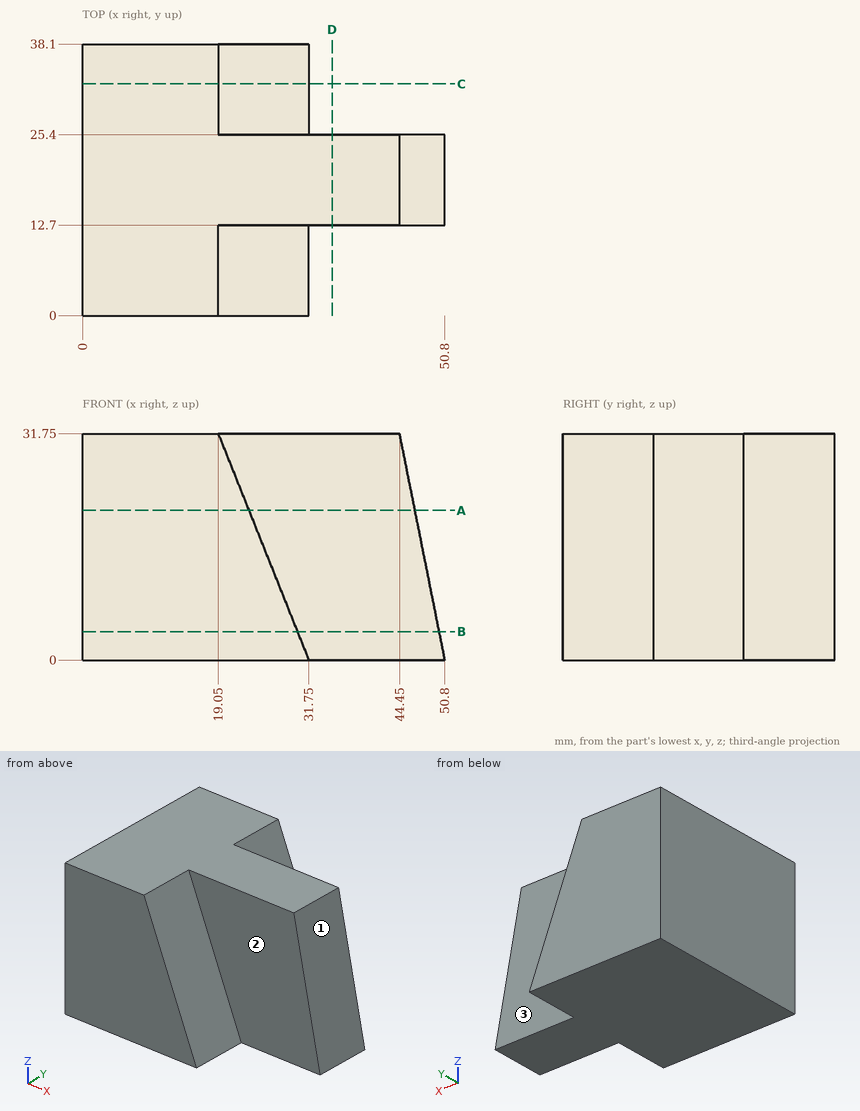
Drawing for the job (mm, zero at the part's lowest x, y, z). A direction names the side the tool comes from. Round coordinates to 2 decimals unless told otherwise and drop trailing zeros. Loops run counter-clockwise (first coordinate to the right, second up) from the corner with the lowest first, then second, coordinate; pieces in that order, holes last. Notation, with made-up numbers: (78.25, -22.75) - (101.25, -22.75) arc R17 cw to (101.25, -5.75) - close; hole circle Ø5 at (-12.5, -2.75). An arc over 180 degrees is marked (long way). Write each question's results on one line, items separated by ' | '.
(1) Saw through at C-C, the plane y = 32.5. List the corners of the cut face in (x, z).
Answer below:
outline: (0, 0) - (31.75, 0) - (19.05, 31.75) - (0, 31.75) - close
(2) Pin check, flat tips, straight feed: pin 1 (1 mm diameter, centred on y = 19, z = 8, fed in from +X); pin 2 (2 mm diameter, centred on x = 33, z = 9.5, fed in from -Y). Stop position of each tip, or through.
Answer below:
pin 1: stops at x = 49.3 | pin 2: stops at y = 12.7
(3) Wall check: L1, parallel to Y at x = 39, z = 27; L2, parallel to X at y = 33.5, z = 28; L3, parallel to X at y = 33, z = 11.5. Give the ranges that are in metal, low to high.
Answer below:
L1: y = 12.7 to 25.4 | L2: x = 0 to 20.55 | L3: x = 0 to 27.15
(4) Saw through at B-B, the plane z = 4. List the corners of the cut face in (x, y).
Answer below:
outline: (0, 0) - (30.15, 0) - (30.15, 12.7) - (50, 12.7) - (50, 25.4) - (30.15, 25.4) - (30.15, 38.1) - (0, 38.1) - close
(5) Saw through at D-D, the plane x = 35. List the corners of the cut face in (y, z), then the cut area to 3 significant figures.
Answer below:
outline: (12.7, 0) - (25.4, 0) - (25.4, 31.75) - (12.7, 31.75) - close | area: 403 mm^2
(6) 3-axis set-ups, long thin cutter, end or side, ignore diameter. For the marked faces 1, 2 and 3: which of +Z, -Z, +X, -X, +Y, -Y reach the whole face in a straight line?
Answer below:
face 1: +Z, +X, +Y, -Y | face 2: +Z, +X, -Y | face 3: +Z, +X, +Y
(7) Saw through at A-A, the plane z = 21. List the corners of the cut face in (x, y), then the cut area to 3 significant figures.
Answer below:
outline: (0, 0) - (23.35, 0) - (23.35, 12.7) - (46.6, 12.7) - (46.6, 25.4) - (23.35, 25.4) - (23.35, 38.1) - (0, 38.1) - close | area: 1,180 mm^2
